Input: dimensioned drawing with shaded views. Units: mm. Origin: part minimum x, y, z. Coordinates: 2 decimals unless noted, no trailing zeros. Loops run counter-clockwise (first coordinate to the right, second up) from the corner with the lowest first, then second, coordinate; pieces in that order, holes last. Notation, with made-up numbers: (28.5, 59) -> (42.5, 59) arc R20 ccw to (42.5, 87) -> close; hole circle Ø2 at (43.25, -31.75). An arc over 180 degrees is marked (long way). Answer as CSV lines item,"result".
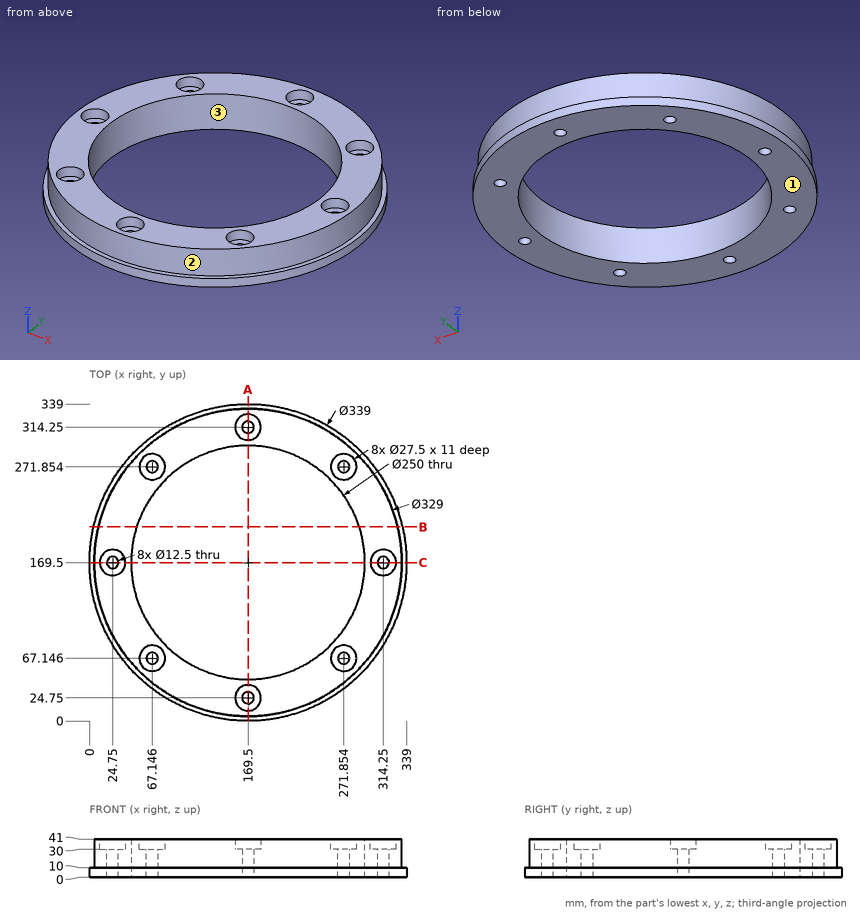
(1) Draft query along X for the marked faces 1, 2 and 3. Return one class per face: released by +X, released by -X, zero draft, split by the parting line, or undercut.
Computed values:
face 1,"zero draft"
face 2,"split by the parting line"
face 3,"undercut"
(2) Material intervals for L1, parallel to Y at x = 169.5, z = 20.5; L2, parallel to Y at x = 65.5, z = 38 (1 decimal); L3, parallel to X at y = 218, z = 15, sorted ascending. Write a range as [from, to].
Computed values:
L1,"[5, 18.5], [31, 44.5], [294.5, 308], [320.5, 334]"
L2,"[42, 53.5], [80.8, 100.2], [238.8, 258.2], [285.5, 297]"
L3,"[12.31, 54.29], [284.71, 326.69]"
(3) Cut plane B-B (y = 207.5). Return the cut outline in (x, z) (1 decimal), then the cut area to 3 significant figures.
Computed values:
outline,"(4.3, 0) -> (50.4, 0) -> (50.4, 41) -> (9.4, 41) -> (9.4, 10) -> (4.3, 10) -> close; (288.6, 0) -> (334.7, 0) -> (334.7, 10) -> (329.6, 10) -> (329.6, 41) -> (288.6, 41) -> close"
area,"3,460 mm^2"
(4) Cut plane A-A (x = 169.5). Return the cut outline in (y, z).
Computed values:
outline,"(0, 0) -> (18.5, 0) -> (18.5, 30) -> (11, 30) -> (11, 41) -> (5, 41) -> (5, 10) -> (0, 10) -> close; (31, 0) -> (44.5, 0) -> (44.5, 41) -> (38.5, 41) -> (38.5, 30) -> (31, 30) -> close; (294.5, 0) -> (308, 0) -> (308, 30) -> (300.5, 30) -> (300.5, 41) -> (294.5, 41) -> close; (320.5, 0) -> (339, 0) -> (339, 10) -> (334, 10) -> (334, 41) -> (328, 41) -> (328, 30) -> (320.5, 30) -> close"
(5) Pin query (flat end, axial travel): pin 1 Ø6 at (x, z) = (60.5, 19) entering from -Y (1 decimal); pin 2 Ø6 at (y, z) = (49, 8.5) entering from +X; pin 3 Ø22 at (x, y) = (24.75, 169.5) entering from +Z. Return the tip coordinate at first contact, or that it passes through.
Computed values:
pin 1,"y = 43.7"
pin 2,"x = 291.66"
pin 3,"z = 30"
